Source: CAD feature listing. Evaluate the final solid. Frame: model axes, mm. Face numbers are marked on the shaded views. A direction names the side the tool comes from. Give positions to 0.01 mm unless a question says otherwise; leave off trailing zeros. Loops run counter-clockwise (first coordinate to the right, second up) from the corner with the lowest first, then second, coordinate; pieces in that order, holes last. Notation, with made-up numbers: M 39.25,-28.5 L 86.25,-28.5 A18 cw 86.25,-20.5 Z; hole C 71,23 d5. An arc over 180 degrees is marked long. Put each result on its own line as item: value.
from build123d import *

# Parameters (mm, degrees)
SKETCH1_R           = 2.5
BOSS_EXTRUDE1_DEPTH = 15
SKETCH2_R           = 12.5
SKETCH2_R_2         = 1.5
CUT_EXTRUDE1_DEPTH  = 10


with BuildPart() as part:
    # Sketch1 → Boss-Extrude1 (new body, symmetric)
    with BuildSketch(Plane(origin=(0, 0, 0), x_dir=(1, 0, 0), z_dir=(0, 1, 0))):
        Circle(SKETCH1_R)
    extrude(amount=BOSS_EXTRUDE1_DEPTH, both=True)

    # Sketch2 → Cut-Extrude1 (cut)
    with BuildSketch(Plane(origin=(0, 15, 0), x_dir=(1, 0, 0), z_dir=(0, 1, 0))):
        Circle(SKETCH2_R)
        Circle(SKETCH2_R_2, mode=Mode.SUBTRACT)
    cut_extrude1 = extrude(amount=-CUT_EXTRUDE1_DEPTH, mode=Mode.SUBTRACT)

    # Mirror1: Cut-Extrude1 across plane
    add(cut_extrude1.mirror(Plane.ZX), mode=Mode.SUBTRACT)


solid = part.part
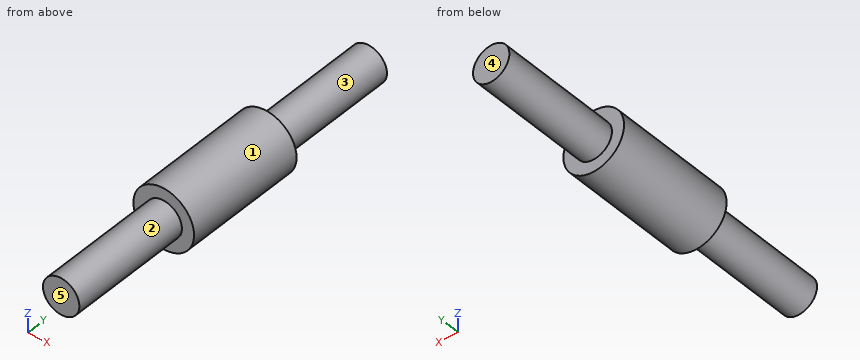
1. Access query for the marked faces 1 and 2. Directions: +Z, -Z, +X, -X, +Y, -Y. A direction counts if a zero-diameter tool reaches every point of the face in a straight line with its end or side. Return the directions, or none.
Found:
face 1: +Y, -Y
face 2: -Y
2. Section query D-D (x = 2). Output: boundary loops of the cut face in (y, z).
Found:
outline: M -5,-1.5 L 5,-1.5 L 5,1.5 L -5,1.5 Z
3. Section query B-B (x = 0). Output: boundary loops of the cut face in (y, z).
Found:
outline: M -15,-1.5 L -5,-1.5 L -5,-2.5 L 5,-2.5 L 5,-1.5 L 15,-1.5 L 15,1.5 L 5,1.5 L 5,2.5 L -5,2.5 L -5,1.5 L -15,1.5 Z
4. Contact query for flat-ended pins moving along their axis: P1, Ø1, axis at x = 1.5, y = -4.5, coming from the +Z side; P2, Ø2, axis at x = -1.5, y = 4, coming from the +Z side; P3, Ø2, axis at x = -0.5, y = 10, coming from the +Z side. Output: stop coordinate, or through.
Found:
P1: z = 2.29
P2: z = 2.45
P3: z = 1.5
5. Section query A-A (z = 0). Output: boundary loops of the cut face in (x, y), plus the area to 3 significant figures.
Found:
outline: M -2.5,-5 L -1.5,-5 L -1.5,-15 L 1.5,-15 L 1.5,-5 L 2.5,-5 L 2.5,5 L 1.5,5 L 1.5,15 L -1.5,15 L -1.5,5 L -2.5,5 Z
area: 110 mm^2
6. Draft query along Y for the marked faces 3, 4 and 5. Return one class per face: pulls with the +Y half, pulls with the -Y half, needs draft (parallel to the pull), parting line crosses it, or undercut.
Found:
face 3: needs draft
face 4: pulls with the +Y half
face 5: pulls with the -Y half
7. Section query C-C (y = 4.5). Output: boundary loops of the cut face in (x, z), plus the area to 3 significant figures.
Found:
outline: C 0,0 d5
area: 19.6 mm^2
8. Material intervals for line 1 (Y direction, x = -2.05, z = 0.2); line 2 (Z direction, x = -0.1, y = 2); line 3 (Z direction, x = 1.3, y = -11), sorted ascending. Write a range as from..to.
Found:
line 1: -5..5
line 2: -2.5..2.5
line 3: -0.75..0.75
